from build123d import *

# Parameters (mm, degrees)
FILLET1_R                   = 0.5
FILLET4_R                   = 0.5
BOSS_EXTRUDE2_START         = 18.65
SKETCH3_R                   = 76
SKETCH3_R_2                 = 46
BOSS_EXTRUDE2_DEPTH         = 18.65
FILLET5_R                   = 5
M12X1_75_TAPPED_HOLE1_D     = 10.2
M12X1_75_TAPPED_HOLE1_DEPTH = 29.25
M12X1_75_TAPPED_HOLE1_TIP   = 3.064389157
SKETCH6_W                   = 6.000865062
SKETCH6_H                   = 152
CUT_EXTRUDE2_DEPTH          = 99


with BuildPart() as part:
    # Sketch1 → Revolve1 (revolve)
    with BuildSketch(Plane(origin=(0, 0, 0), x_dir=(1, 0, 0), z_dir=(0, 1, 0)), mode=Mode.PRIVATE) as revolve1_sk:
        with BuildLine():
            Line((0.595225647, 30), (2.595225647, 30))
            Line((2.595225647, 30), (2.595225647, 40))
            ThreePointArc((2.595225647, 40), (3.181012085, 41.414213562), (4.595225647, 42))
            Line((4.595225647, 42), (6.595225647, 42))
            Line((6.595225647, 42), (6.595225647, 47))
            Line((6.595225647, 47), (3.744360585, 47))
            Line((3.744360585, 47), (3.744360585, 76))
            Line((3.744360585, 76), (-2.255639415, 76))
            Line((-2.255639415, 76), (-2.255639415, 49))
            ThreePointArc((-2.255639415, 49), (-3.134319072, 46.878679656), (-5.255639415, 46))
            Line((-5.255639415, 46), (-6.404774353, 46))
            Line((-6.404774353, 46), (-6.404774353, 36))
            Line((-6.404774353, 36), (0.595225647, 36))
            Line((0.595225647, 36), (0.595225647, 30))
        make_face()
    revolve(revolve1_sk.sketch.rotate(Axis((0, 0, 0), (1, 0, 0)), 180), axis=Axis((0, 0, 0), (1, 0, 0)))

    # Fillet1
    fillet1_edges = [part.edges().sort_by_distance(p)[0] for p in [
        (-6.404774353, 0, -36),
    ]]
    fillet(fillet1_edges, radius=FILLET1_R)

    # Fillet4
    fillet4_edges = [part.edges().sort_by_distance(p)[0] for p in [
        (6.595225647, 0, -47),
    ]]
    fillet(fillet4_edges, radius=FILLET4_R)

    # Sketch3 → Boss-Extrude2 (add)
    with BuildSketch(Plane.ZY.offset(2.255639415).offset(BOSS_EXTRUDE2_START)):
        Circle(SKETCH3_R)
        with Locations(Location((0, 0, 0), (0, 0, 180))):
            Circle(SKETCH3_R_2, mode=Mode.SUBTRACT)
    extrude(amount=-BOSS_EXTRUDE2_DEPTH)

    # Fillet5
    fillet5_edges = [part.edges().sort_by_distance(p)[0] for p in [
        (3.744360585, 0, -76),
    ]]
    fillet(fillet5_edges, radius=FILLET5_R)

    # M12x1.75 Tapped Hole1
    with Locations(Plane(origin=(3.744360585, 0, 0), x_dir=(0, 0, -1), z_dir=(1, 0, 0))):
        with Locations((0, 58.75), (50.878992472, 29.375), (50.878992472, -29.375), (0, -58.75), (-50.878992472, -29.375), (-50.878992472, 29.375)):
            Hole(M12X1_75_TAPPED_HOLE1_D / 2, depth=M12X1_75_TAPPED_HOLE1_DEPTH)
            with Locations((0, 0, -(M12X1_75_TAPPED_HOLE1_DEPTH + M12X1_75_TAPPED_HOLE1_TIP / 2))):  # 118° drill point
                Cone(0, M12X1_75_TAPPED_HOLE1_D / 2, M12X1_75_TAPPED_HOLE1_TIP, mode=Mode.SUBTRACT)

    # Sketch6 → Cut-Extrude2 (cut, symmetric)
    with BuildSketch(Plane(origin=(0, 0, 0), x_dir=(1, 0, 0), z_dir=(0, 1, 0))):
        with Locations((-17.905206884, 0)):
            Rectangle(SKETCH6_W, SKETCH6_H)
    extrude(amount=CUT_EXTRUDE2_DEPTH, both=True, mode=Mode.SUBTRACT)


solid = part.part
Source: CAD feature listing. Evaluate the final solid. Frame: model axes, mm. A direction names the side the tool comes from. Give positions to 0.01 mm unless a question says otherwise; leave off trailing zeros. Order: outer loops, then holes, each group sorted by start corner. A loop starts at its lowest first (then second) coordinate and runs counter-clockwise, first axis right, second up. Notation, with made-up numbers: (74.25, 85.25) -> (122.25, 85.25) arc R19 ccw to (122.25, 122.25) -> close; hole circle Ø9 at (18.25, -15.75). An arc over 180 degrees is marked (long way). Write item = value, one per line.
Q1. Material intervals for line 1 (Y direction, x = -3, z = 0); line 2 (Y direction, x = -12.5, z = 54.5); line 3 (Y direction, x = -0.25, z = 51), sorted ascending. Write a range as from..to.
Data:
line_1 = -76..-63.85, -53.65..-36, 36..53.65, 63.85..76
line_2 = -52.97..-32.97, -25.78..25.78, 32.97..52.97
line_3 = -56.21..-34.47, -24.28..24.28, 34.47..56.21
Q2. Pull-direction query (Z, two-part tool) for faces 4 (the face through (-8.176, -67.425, 35.069)), 5 (the face through (-5.7, -53.7, -0.7)), 6 (the face through (6.595, 24, 35)), 7 (the face through (-10.71, -45.61, 5.99)); classes: released by +Z, released by -Z, zero draft, split by the parting line, or undercut.
Data:
face_4 = split by the parting line
face_5 = undercut
face_6 = zero draft
face_7 = undercut
Q3. Cut plane B-B, the plane z = 0. State how many separate pieces and enclosed holes the cut face has, and give its area (3 significant figures).
Data:
separate_pieces = 4
enclosed_holes = 0
area = 971 mm^2
Q4. Set-up query: faces 1 (the face through (0.595, -27, -14)), 2 (the face through (4.9, -46.6, -6.12)), 3 (the face through (-5.711, 26.272, 46.832)). Return all of +Z, -Z, +X, -X, +Y, -Y with unobstructed straight access to the full face (end or side cutting, diameter ignored); none if empty.
Data:
face_1 = -X
face_2 = +X
face_3 = +X, -X
Q5. Cut plane C-C, the plane x = -11. Output: boundary loops of the cut face in (y, z) (3 decimals).
Data:
outline = circle Ø152 at (0, 0); hole circle Ø10.2 at (-58.75, 0); hole circle Ø92 at (0, 0); hole circle Ø10.2 at (-29.375, -50.879); hole circle Ø10.2 at (-29.375, 50.879); hole circle Ø10.2 at (29.375, -50.879); hole circle Ø10.2 at (29.375, 50.879); hole circle Ø10.2 at (58.75, 0)
Q6. Pin query (flat end, axial travel): pin 1 (13.5 mm diameter, centred on y = -58.75, z = 0, fed in from +X); pin 2 (3 mm diameter, centred on x = 1.5, z = -41.5, fed in from +Y); pin 3 (9 mm diameter, centred on y = 29.38, z = -50.88, fed in from +X); pin 4 (6 mm diameter, centred on x = -11.5, z = -47, fed in from -Y). Return the tip coordinate at first contact, or that it passes through.
Data:
pin_1 = 3.74
pin_2 = 64.01
pin_3 = through
pin_4 = -61.97
